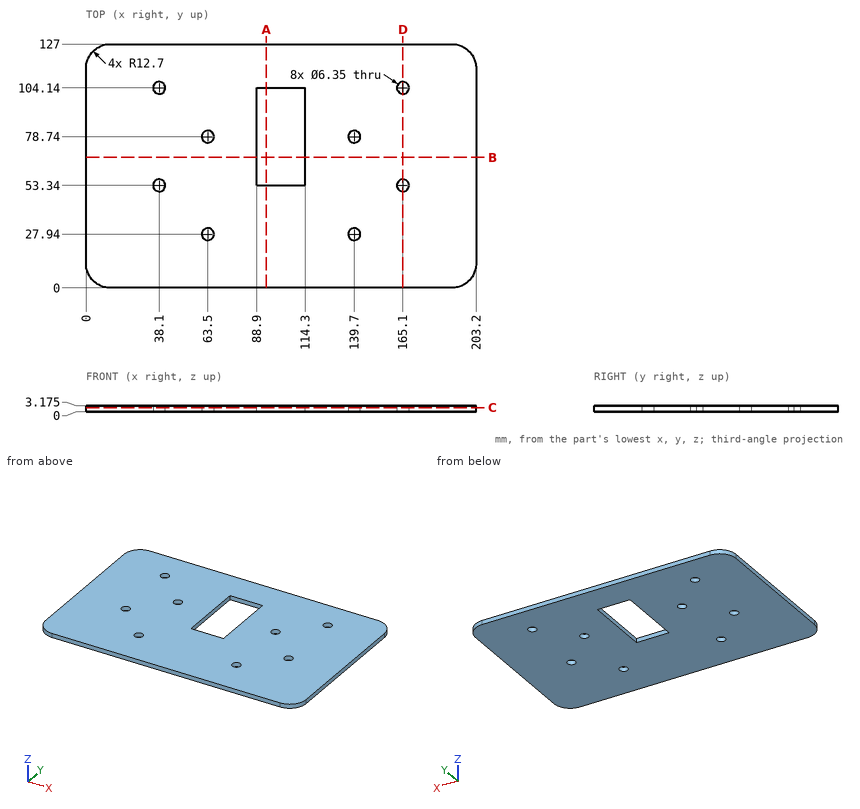
Check sheet for the drawn part. Datum: minimum x, y, z corner. Units: mm. Give positions to 0.01 mm unless a question says otherwise; leave off trailing zeros. Order: outer loops, then holes, each group sorted by start corner. A loop starts at its lowest first (then second) coordinate and runs counter-clockwise, first axis right, second up. Notation, with made-up numbers: (-35.75, -3.5) - (9.25, -3.5) arc R22 ccw to (9.25, 2.5) - close; hole circle Ø6 at (82.5, 18). An arc over 180 degrees is marked (long way). Write item = value, one per line. Start each with the question number.
1) Section check C-C (z = 2.3). Count the separate pieces of the cut face and the enclosed holes in it, then the cut area to 3 significant figures.
2) Section check D-D (x = 165.1). Enter the section's corners in (y, z) (3 decimals).
3) Section check B-B (y = 68). Enter the section's corners in (x, z) (3 decimals), then the cut area to 3 significant figures.
4) Section check A-A (x = 94). Enter the section's corners in (y, z) (3 decimals), then the cut area to 3 significant figures.
5) Scan lines: L1, parallel to Y at x = 38.1, z = 0.85 (3 decimals); L2, parallel to Y at x = 139.7, z = 0.8 (3 decimals); L3, parallel to X at y = 60, z = 0.45. Record each from-to range of solid material in increasing order.
Geometry check:
q1.separate_pieces = 1
q1.enclosed_holes = 9
q1.area = 24,100 mm2
q2.outline = (0, 0) - (50.165, 0) - (50.165, 3.175) - (0, 3.175) - close; (56.515, 0) - (100.965, 0) - (100.965, 3.175) - (56.515, 3.175) - close; (107.315, 0) - (127, 0) - (127, 3.175) - (107.315, 3.175) - close
q3.outline = (0, 0) - (88.9, 0) - (88.9, 3.175) - (0, 3.175) - close; (114.3, 0) - (203.2, 0) - (203.2, 3.175) - (114.3, 3.175) - close
q3.area = 565 mm2
q4.outline = (0, 0) - (53.34, 0) - (53.34, 3.175) - (0, 3.175) - close; (104.14, 0) - (127, 0) - (127, 3.175) - (104.14, 3.175) - close
q4.area = 242 mm2
q5.L1 = 0 to 50.165, 56.515 to 100.965, 107.315 to 127
q5.L2 = 0 to 24.765, 31.115 to 75.565, 81.915 to 127
q5.L3 = 0 to 88.9, 114.3 to 203.2
